from build123d import *

# Parameters (mm, degrees)
SKETCH1_W           = 38.1
SKETCH1_H           = 31.75
BOSS_EXTRUDE1_DEPTH = 76.2
BOSS_EXTRUDE1_DRAFT = -5
SKETCH3_W           = 31.75
SKETCH3_H           = 22.225
CUT_EXTRUDE1_DEPTH  = 84.5219177
CUT_EXTRUDE1_DRAFT  = 5
FILLET1_R           = 2.54


with BuildPart() as part:
    # Sketch1 → Boss-Extrude1 (with draft: the straight prism first)
    with BuildSketch(Plane(origin=(0, 0, 0), x_dir=(1, 0, 0), z_dir=(0, 1, 0))):
        Rectangle(SKETCH1_W, SKETCH1_H)
    extrude(amount=BOSS_EXTRUDE1_DEPTH)
    # Boss-Extrude1: the draft: its side faces are tilted about the plane it starts from
    boss_extrude1_sides = [part.faces().sort_by_distance(p)[0] for p in [
        (0, 38.1, 15.875),
        (19.05, 38.1, 0),
        (0, 38.1, -15.875),
        (-19.05, 38.1, 0),
    ]]
    draft(boss_extrude1_sides, Plane(origin=(0, 0, 0), x_dir=(1, 0, 0), z_dir=(0, 1, 0)), BOSS_EXTRUDE1_DRAFT)


with BuildPart() as cut_extrude1_tool:
    # Sketch3 → Cut-Extrude1 (with draft: the straight prism first)
    with BuildSketch(Plane.XZ):
        Rectangle(SKETCH3_W, SKETCH3_H)
    extrude(amount=-CUT_EXTRUDE1_DEPTH)
    # Cut-Extrude1: the draft: its side faces are tilted about the plane it starts from
    cut_extrude1_sides = [cut_extrude1_tool.faces().sort_by_distance(p)[0] for p in [
        (0, 42.26095885, -11.1125),
        (15.875, 42.26095885, 0),
        (0, 42.26095885, 11.1125),
        (-15.875, 42.26095885, 0),
    ]]
    draft(cut_extrude1_sides, Plane.XZ, CUT_EXTRUDE1_DRAFT)


with BuildPart() as part_1:
    add(part.part)

    # Cut-Extrude1: cut by cut_extrude1_tool
    add(cut_extrude1_tool.part, mode=Mode.SUBTRACT)

    # Fillet1
    fillet1_edges = [part_1.edges().sort_by_distance(p)[0] for p in [
        (22.38331808, 38.1, 19.20831808),
        (-22.38331808, 38.1, 19.20831808),
        (-22.38331808, 38.1, -19.20831808),
        (22.38331808, 38.1, -19.20831808),
    ]]
    fillet(fillet1_edges, radius=FILLET1_R)


solid = part_1.part
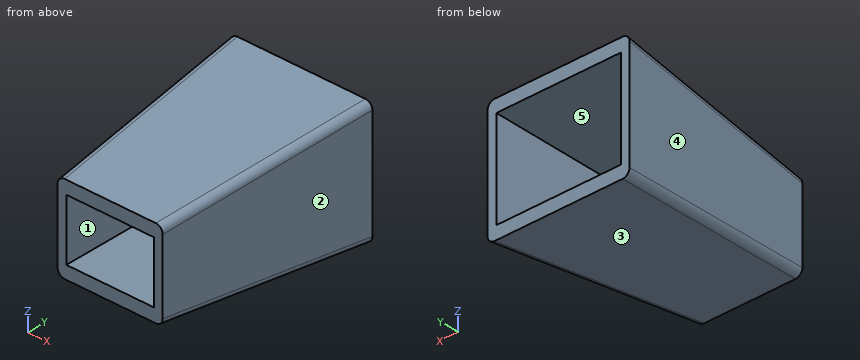
Work out the finished part from the listing and answer in its coordinate system (mm). Face numbers are marked on the shaded views. A direction names the side the tool comes from. Give positions to 0.01 mm unless a question says otherwise; leave off trailing zeros. Write each loop counter-clockwise with the first axis right and the second up, starting at its lowest first coordinate (ties: lowest second). Pieces come first, ordered by that corner, then holes. Notation, with made-up numbers: (2.5, 72) - (16.5, 72) arc R20 cw to (16.5, 110) - close; hole circle Ø3 at (-38, 38). An arc over 180 degrees is marked (long way). One line per item, written item: value. Start each with the question number.
1. Given pin 1 (5 mm diameter, centred on x = -11.5, y = 67, fed in from -Z); pin 2 (6 mm diameter, centred on x = -2, y = 56.5, fed in from +Z); pin 3 (8 mm diameter, centred on x = 12, y = 34, fed in from +Z); pin 4 (2 mm diameter, centred on x = -0.5, z = -16.5, fed in from -Y), each flat-ended and moving along its own axis, determine where each tip first touches the part or whether it passes through.
2. For the marked faces 1 and 2, determine the directions among +Z, -Z, +X, -X, +Y, -Y from which every point of the face is accessible in a straight line to the end or side of a thin tool.
3. For a pull along Z with two mould halves and no side action, classify the marked faces 3, 4 and 5 as +Z half, -Z half, draft (parallel to the pull), parting line (faces both ways), or undercut.
4. Find section B-B (x = -6). Write down the section's boundary in (y, z) (1 decimal), then the cut area to 3 significant figures.
5. Find section A-A (z = 0.5). Write down the section's boundary in (x, y) (3 decimals).
6. Consider probe 1 along X at (y, z) = (22, -4); probe 2 along Z at (x, y) = (-16, 19.5); probe 3 along Z at (x, y) = (-3, 18). Determine where each line is inside the solid, lowest interval first.
Geometry results:
1. pin 1: z = -21.96
1. pin 2: z = 21.08
1. pin 3: z = 19.2
1. pin 4: y = 0
2. face 1: +Y
2. face 2: +Z, -Z, +X, -Y
3. face 3: -Z half
3. face 4: draft
3. face 5: undercut
4. outline: (0, -15.9) - (76.2, -22.5) - (76.2, -17.8) - (0, -11.1) - close; (0, 11.1) - (76.2, 17.8) - (76.2, 22.5) - (0, 15.9) - close
4. area: 726 mm2
5. outline: (-25.717, 76.2) - (-19.05, 0) - (-15.875, 0) - (-22.542, 76.2) - close; (15.875, 0) - (19.05, 0) - (25.717, 76.2) - (22.542, 76.2) - close
6. probe 1: -20.97 to -17.8, 17.8 to 20.97
6. probe 2: -17.58 to -12.82, 12.82 to 17.58
6. probe 3: -17.45 to -12.69, 12.69 to 17.45
